from build123d import *

# Parameters (mm, degrees)
SKETCH_W        = 70
SKETCH_H        = 70
PAD_DEPTH       = 2
SKETCH001_W     = 49
SKETCH001_H     = 49
PAD001_DEPTH    = 28
SKETCH002_W     = 45
SKETCH002_H     = 45
POCKET_DEPTH    = 28
SKETCH003_W     = 16
SKETCH003_H     = 11.09878
POCKET001_DEPTH = 18
SKETCH004_W     = 45
SKETCH004_H     = 2
PAD002_DEPTH    = 10
SKETCH005_W     = 41.4
SKETCH005_H     = 15.4
PAD003_DEPTH    = 4
SKETCH006_W     = 39
SKETCH006_H     = 13
POCKET002_DEPTH = 5
SKETCH007_W     = 23
SKETCH007_H     = 7
POCKET003_DEPTH = 1.001
POCKET004_DEPTH = 5
SKETCH009_R     = 1.6
POCKET005_DEPTH = 59.501
FILLET_R        = 15
SKETCH010_R     = 2
PAD004_DEPTH    = 13


with BuildPart() as part:
    # Sketch → Pad (new body)
    with BuildSketch(Plane.XY):
        Rectangle(SKETCH_W, SKETCH_H)
        with BuildLine():
            ThreePointArc((27.608372, -4.666667), (28, 0), (27.608372, 4.666667))
            ThreePointArc((31.552426, 5.333333), (29.247066, 6.972027), (27.608372, 4.666667))
            ThreePointArc((31.552426, -5.333333), (32, 0), (31.552426, 5.333333))
            ThreePointArc((27.608372, -4.666667), (29.247066, -6.972027), (31.552426, -5.333333))
        make_face(mode=Mode.SUBTRACT)
        with BuildLine():
            ThreePointArc((-27.608372, 4.666667), (-28, 0), (-27.608372, -4.666667))
            ThreePointArc((-31.552426, -5.333333), (-29.247066, -6.972027), (-27.608372, -4.666667))
            ThreePointArc((-31.552426, 5.333333), (-32, 0), (-31.552426, -5.333333))
            ThreePointArc((-27.608372, 4.666667), (-29.247066, 6.972027), (-31.552426, 5.333333))
        make_face(mode=Mode.SUBTRACT)
    extrude(amount=PAD_DEPTH)

    # Sketch001 (on Face14 of Pad) → Pad001 (join)
    with BuildSketch(Plane.XY.offset(2)):
        Rectangle(SKETCH001_W, SKETCH001_H)
    extrude(amount=PAD001_DEPTH)

    # Sketch002 (on Face19 of Pad001) → Pocket (cut)
    with BuildSketch(Plane.XY.offset(30)):
        Rectangle(SKETCH002_W, SKETCH002_H)
    extrude(amount=-POCKET_DEPTH, mode=Mode.SUBTRACT)

    # Sketch003 (on Face19 of Pocket) → Pocket001 (cut)
    with BuildSketch(Plane.XY.offset(30)):
        with Locations((12.5, -23.806966)):
            Rectangle(SKETCH003_W, SKETCH003_H)
    extrude(amount=-POCKET001_DEPTH, mode=Mode.SUBTRACT)

    # Sketch004 (on Face27 of Pocket001) → Pad002 (join)
    with BuildSketch(Plane.XY.offset(2)):
        with Locations((0, -0.5)):
            Rectangle(SKETCH004_W, SKETCH004_H)
    extrude(amount=PAD002_DEPTH)

    # Sketch005 (on Face27 of Pad002) → Pad003 (join)
    with BuildSketch(Plane.XY.offset(2)):
        with Locations((0, -12)):
            Rectangle(SKETCH005_W, SKETCH005_H)
    extrude(amount=PAD003_DEPTH)

    # Sketch006 (on Face36 of Pad003) → Pocket002 (cut)
    with BuildSketch(Plane.XY.offset(6)):
        with Locations((0, -12)):
            Rectangle(SKETCH006_W, SKETCH006_H)
    extrude(amount=-POCKET002_DEPTH, mode=Mode.SUBTRACT)

    # Sketch007 (on Face41 of Pocket002) → Pocket003 (cut, through all)
    with BuildSketch(Plane.XY.offset(1)):
        with Locations((0, -11)):
            Rectangle(SKETCH007_W, SKETCH007_H)
    extrude(amount=-POCKET003_DEPTH, mode=Mode.SUBTRACT)

    # Sketch008 (on Face37 of Pocket003) → Pocket004 (cut)
    with BuildSketch(Plane.XY.offset(2)):
        with BuildLine():
            Line((-11, 15.5), (-11, 2.5))
            ThreePointArc((-11, 2.5), (-10, 1.5), (-9, 2.5))
            Line((-9, 15.5), (-9, 2.5))
            ThreePointArc((-9, 15.5), (-10, 16.5), (-11, 15.5))
        make_face()
        with BuildLine():
            Line((-7, 15.5), (-7, 2.5))
            ThreePointArc((-7, 2.5), (-6, 1.5), (-5, 2.5))
            Line((-5, 15.5), (-5, 2.5))
            ThreePointArc((-5, 15.5), (-6, 16.5), (-7, 15.5))
        make_face()
        with BuildLine():
            Line((-3, 15.5), (-3, 2.5))
            ThreePointArc((-3, 2.5), (-2, 1.5), (-1, 2.5))
            Line((-1, 15.5), (-1, 2.5))
            ThreePointArc((-1, 15.5), (-2, 16.5), (-3, 15.5))
        make_face()
        with BuildLine():
            Line((1, 15.5), (1, 2.5))
            ThreePointArc((1, 2.5), (2, 1.5), (3, 2.5))
            Line((3, 15.5), (3, 2.5))
            ThreePointArc((3, 15.5), (2, 16.5), (1, 15.5))
        make_face()
        with BuildLine():
            Line((5, 15.5), (5, 2.5))
            ThreePointArc((5, 2.5), (6, 1.5), (7, 2.5))
            Line((7, 15.5), (7, 2.5))
            ThreePointArc((7, 15.5), (6, 16.5), (5, 15.5))
        make_face()
        with BuildLine():
            Line((9, 15.5), (9, 2.5))
            ThreePointArc((9, 2.5), (10, 1.5), (11, 2.5))
            Line((11, 15.5), (11, 2.5))
            ThreePointArc((11, 15.5), (10, 16.5), (9, 15.5))
        make_face()
    extrude(amount=-POCKET004_DEPTH, mode=Mode.SUBTRACT)

    # Sketch009 (on Face45 of Pocket004) → Pocket005 (cut, through all)
    with BuildSketch(Plane.XZ.offset(24.5)):
        with Locations((0, 25)):
            Circle(SKETCH009_R)
    extrude(amount=-POCKET005_DEPTH, mode=Mode.SUBTRACT)

    # Fillet
    fillet_edges = [part.edges().sort_by_distance(p)[0] for p in [
        (-35, 35, 1),
        (35, 35, 1),
        (35, -35, 1),
        (-35, -35, 1),
    ]]
    fillet(fillet_edges, radius=FILLET_R)

    # Sketch010 (on Face52 of Fillet) → Pad004 (join)
    with BuildSketch(Plane.XY.offset(2)):
        with Locations((22.5, 22.5)):
            Circle(SKETCH010_R)
        with Locations((-22.5, 22.5)):
            Circle(SKETCH010_R)
        with Locations((22.5, 0.6)):
            Circle(SKETCH010_R)
        with Locations((0, -22.5)):
            Circle(SKETCH010_R)
        with Locations((-22.5, -22.5)):
            Circle(SKETCH010_R)
    extrude(amount=PAD004_DEPTH)


solid = part.part
Verification items for the finished model (mm, model axes). A direction names the side the tool comes from. Round coordinates to 2 decimals unless told otherwise and drop trailing zeros. Loops run counter-clockwise (first coordinate to the right, second up) from the corner with the lowest first, then second, coordinate; pieces in that order, holes last. Notation, with made-up numbers: (78, 47) - (91, 47) arc R19 ccw to (91, 83) - close; hole circle Ø10 at (72.5, 44.25). An arc over 180 degrees is marked (long way). Answer in a Markdown table with one row per item. Add a question column.
Q1. Release check for a two-part mould opening along Y. For faces 1 (the face through (5, 26, 2)), 2 (the face through (29.204, -6.964, 0.986)) record: pulls with the +Y half, pulls with the -Y half, needs draft (parallel to the pull), parting line crosses it, or undercut.
Q2. Section check B-B on z = 4. Enter the section's corners in (x, y), plus the area to 3 significant figures.
Q3. Gauge pin test, flat ends, axial feed: pin 1 (10 mm diameter, centred on x = 10, y = 0, fed in from +Z); pin 2 (1.5 mm diameter, centred on x = 2, z = 21.5, fed in from -Y); pin 3 (0.6 mm diameter, centred on x = -22, y = -21, fed in from +Z). Record the tip position at first contact, or that the pin passes through.
Q4. Section check A-A on x = -6. State how many separate pieces and enclosed holes the cut face has, plus the area to 3 significant figures.
Q5. Section check D-D on x = -17. Enter the section's corners in (y, z), plus the area to 3 significant figures.
Q6. Material ranges on line 1 (Y direction, x = -3.5, z = 2.75); line 2 (X direction, y = 2, z = 16.25); line 3 (Z direction, x = 0, y = 23), recorded low to high.
Q7. Tool access check on faces 3 (the face through (-1.27, -23.51, 24.03)), 4 (the face through (-2, 1.5, 1)), 5 (the face through (22, 1, 15)). Record the directions out of +Z, -Z, +X, -X, +Y, -Y that give a thin tool (end or side, any length) a straight path to the whole face; none if there is none.
Q8. Section check C-C on y = -12. Enter the section's corners in (x, z), plus the area to 3 significant figures.
Found:
| question | item | result |
|---|---|---|
| 1 | face 1 | needs draft |
| 1 | face 2 | undercut |
| 2 | outline | (-24.5, -24.5) - (24.5, -24.5) - (24.5, 24.5) - (-24.5, 24.5) - close; (-20.7, -19.7) - (20.7, -19.7) - (20.7, -4.3) - (-20.7, -4.3) - close; hole (-22.5, -20.5) arc R2 cw to (-20.5, -22.5) - (-2, -22.5) arc R2 cw to (2, -22.5) - (22.5, -22.5) - (22.5, -1.5) - (-22.5, -1.5) - close; hole (-22.5, 0.5) - (20.5, 0.5) arc R2 cw to (22.5, 2.6) - (22.5, 20.5) arc R2 cw to (20.5, 22.5) - (-20.5, 22.5) arc R2 cw to (-22.5, 20.5) - close; hole (-19.5, -18.5) - (19.5, -18.5) - (19.5, -5.5) - (-19.5, -5.5) - close |
| 2 | area | 616 mm² |
| 3 | pin 1 | stops at z = 12 |
| 3 | pin 2 | stops at y = -24.5 |
| 3 | pin 3 | stops at z = 15 |
| 4 | separate pieces | 3 |
| 4 | enclosed holes | 0 |
| 4 | area | 232 mm² |
| 5 | outline | (-35, 0) - (35, 0) - (35, 2) - (24.5, 2) - (24.5, 30) - (22.5, 30) - (22.5, 2) - (0.5, 2) - (0.5, 12) - (-1.5, 12) - (-1.5, 2) - (-4.3, 2) - (-4.3, 6) - (-5.5, 6) - (-5.5, 1) - (-18.5, 1) - (-18.5, 6) - (-19.7, 6) - (-19.7, 2) - (-22.5, 2) - (-22.5, 30) - (-24.5, 30) - (-24.5, 2) - (-35, 2) - close |
| 5 | area | 269 mm² |
| 6 | line 1 | y = -24.5 to -22.5, -19.7 to -18.5, -5.5 to -4.3, -1.5 to 0.5, 22.5 to 24.5 |
| 6 | line 2 | x = -24.5 to -22.5, 22.5 to 24.5 |
| 6 | line 3 | z = 0 to 23.4, 26.6 to 30 |
| 7 | face 3 | +Y, -Y |
| 7 | face 4 | +Z, -Z |
| 7 | face 5 | +Z |
| 8 | outline | (-35, 0) - (-11.5, 0) - (-11.5, 1) - (-19.5, 1) - (-19.5, 6) - (-20.7, 6) - (-20.7, 2) - (-22.5, 2) - (-22.5, 30) - (-24.5, 30) - (-24.5, 2) - (-35, 2) - close; (11.5, 0) - (35, 0) - (35, 2) - (24.5, 2) - (24.5, 30) - (22.5, 30) - (22.5, 2) - (20.7, 2) - (20.7, 6) - (19.5, 6) - (19.5, 1) - (11.5, 1) - close |
| 8 | area | 200 mm² |
